```python
from build123d import *

# Parameters (mm, degrees)
BOSS_EXTRUDE1_DEPTH = 12
FILLET3_R           = 1


with BuildPart() as part:
    # Sketch1 → Boss-Extrude1 (new body)
    with BuildSketch(Plane.XY):
        Polygon((0, 0), (0, 12), (12, 12), (12, 0), (10, 0), (10, 10), (2, 10), (2, 0), align=None)
    extrude(amount=BOSS_EXTRUDE1_DEPTH)

    # Fillet3
    fillet3_edges = [part.edges().sort_by_distance(p)[0] for p in [
        (2, 5, 12),
        (0, 6, 12),
        (12, 6, 12),
        (10, 5, 12),
        (6, 10, 12),
        (6, 12, 12),
        (0, 12, 6),
        (12, 12, 6),
        (12, 6, 0),
        (6, 12, 0),
        (0, 6, 0),
        (10, 5, 0),
        (6, 10, 0),
        (2, 5, 0),
    ]]
    fillet(fillet3_edges, radius=FILLET3_R - 0.0001)  # a hair under: the kernel refuses the full size


solid = part.part
```
Input: part model. Units: mm. Frame: model coordinates. A direction names the side the tool comes from. Coordinates: 2 decimals unless noted, no trailing zeros. Order: outer loops, then holes, each group sorted by start corner. A loop starts at its lowest first (then second) coordinate and runs counter-clockwise, first axis right, second up. Notation, with made-up numbers: (20, 63.5) - (78, 63.5) arc R25 cw to (78, 99.5) - close; hole circle Ø11 at (64, 42). An arc over 180 degrees is marked (long way). Return JSON: item names as keys, results as strings.
Q1. Cut plane B-B (z = 5). Return loops of the section in (x, y), then the cut area to 3 significant figures.
The answers:
{"outline": "(0, 0) - (2, 0) - (2, 10) - (10, 10) - (10, 0) - (12, 0) - (12, 11) arc R1 ccw to (11, 12) - (1, 12) arc R1 ccw to (0, 11) - close", "area": "63.6 mm2"}
Q2. First-contact query: pin 1 (4 mm diameter, centred on x = 3.5, y = 4, fed in from -Z). Flat tip, straight axial feed; report the tip coordinate or a pass-through.
The answers:
{"pin 1": "stops at z = 0.13"}
Q3. Access query for faces 5 (the cylindrical face through (6.07, 11.715, 11.699)), 6 (the cylindrical face through (5.93, 10.285, 0.301)), 7 (the flat face through (10, 5, 6)), 8 (the cylindrical face through (10.285, 5.577, 11.699)). Directions: +Z, -Z, +X, -X, +Y, -Y. A direction counts if a zero-diameter tool reaches every point of the face in a straight line with its end or side. Return the directions, or none.
The answers:
{"face 5": "+Z, +X, -X, +Y", "face 6": "-Z, -Y", "face 7": "+Z, -Z, -Y", "face 8": "+Z, -Y"}
Q4. Ray query, probe 1 along X at (y, z) = (3, 1.25); probe 2 along Y at (x, z) = (7, 5.5); probe 3 along X at (y, z) = (11.5, 1.25). Return the intervals inside material, ascending.
The answers:
{"probe 1": "x = 0 to 2, 10 to 12", "probe 2": "y = 10 to 12", "probe 3": "x = 0.13 to 11.87"}
Q5. Draft query along X for faces 1 (the cylindrical face through (11.699, 11.715, 6.07)), 2 (the cylindrical face through (5.93, 10.285, 11.699)), 3 (the cylindrical face through (1.715, 5.423, 11.699)), 4 (the cylindrical face through (0.285, 11.699, 6.07)). Return one class per face: +X half, -X half, draft (parallel to the pull), parting line (faces both ways), or undercut.
The answers:
{"face 1": "+X half", "face 2": "undercut", "face 3": "undercut", "face 4": "-X half"}
Q6. Cut plane D-D (y = 11.25). Return loops of the section in (x, z).
The answers:
{"outline": "(0.03, 1) arc R0.97 ccw to (1, 0.03) - (11, 0.03) arc R0.97 ccw to (11.97, 1) - (11.97, 11) arc R0.97 ccw to (11, 11.97) - (1, 11.97) arc R0.97 ccw to (0.03, 11) - close"}
